Verification items for the finished model (mm, model axes). A direction names the side the tool comes from. Give positions to 0.01 mm unless a question says otherwise; leave off trailing zeros. Loops run counter-clockwise (first coordinate to the right, second up) from the corner with the lowest first, then second, coordinate; pieces in that order, holes last. Notation, with made-up numbers: M -25,-19 L 7,-19 A16 cw 7,7 Z; hole C 53,-38 d9. An arc over 180 degrees is marked long. Put each result on its own line as item: value. Start each with the question number.
from build123d import *

# Parameters (mm, degrees)
SKETCH1_R           = 4.60375
BOSS_EXTRUDE1_DEPTH = 127
SKETCH3_R           = 1.249999967
CUT_EXTRUDE3_DEPTH  = 190.290136172
SKETCH4_R           = 1.1
CUT_EXTRUDE4_DEPTH  = 189.880695817
SKETCH5_W           = 5.08
SKETCH5_H           = 127
BOSS_EXTRUDE2_DEPTH = 50.8
SKETCH6_R           = 0.899999978
CUT_EXTRUDE5_DEPTH  = 5.08
SKETCH7_W           = 6.432611175
SKETCH7_H           = 24.280435839
SKETCH7_W_2         = 25.4
SKETCH7_H_2         = 5.08
SKETCH7_W_3         = 7.534248642
SKETCH7_H_3         = 19.188789511
CUT_EXTRUDE6_DEPTH  = 196.180089282
FILLET1_R           = 5.08
SKETCH8_W           = 43.18
SKETCH8_H           = 7.62
BOSS_EXTRUDE3_DEPTH = 62.23
FILLET2_R           = 5.08


with BuildPart() as part:
    # Sketch1 → Boss-Extrude1 (new body)
    with BuildSketch(Plane.XY):
        with BuildLine():
            Line((-0.467721946, 0.970453027), (-0.467721946, -10.459546973))
            Line((-0.467721946, -10.459546973), (139.232278054, -10.459546973))
            Line((139.232278054, -10.459546973), (139.232278054, 0.970453027))
            ThreePointArc((139.232278054, 0.970453027), (132.882278054, 7.320453027), (126.532278054, 0.970453027))
            Line((126.532278054, 0.970453027), (126.532278054, -5.379546973))
            Line((126.532278054, -5.379546973), (12.232278054, -5.379546973))
            Line((12.232278054, -5.379546973), (12.232278054, 0.970453027))
            ThreePointArc((12.232278054, 0.970453027), (5.882278054, 7.320453027), (-0.467721946, 0.970453027))
        make_face()
        with Locations((5.882278054, 0.970453027)):
            Circle(SKETCH1_R, mode=Mode.SUBTRACT)
        with Locations((132.882278054, 0.970453027)):
            Circle(SKETCH1_R, mode=Mode.SUBTRACT)
    extrude(amount=BOSS_EXTRUDE1_DEPTH)

    # Sketch3 → Cut-Extrude3 (cut, through all)
    with BuildSketch(Plane.XZ.offset(10.459546973)):
        with Locations(Location((101.132278054, 81.883033078, 0), (0, 0, 270))):
            Circle(SKETCH3_R)
        with Locations(Location((43.132278054, 81.883033078, 0), (0, 0, 270))):
            Circle(SKETCH3_R)
        with Locations(Location((43.132278054, 32.883033078, 0), (0, 0, 270))):
            Circle(SKETCH3_R)
        with Locations(Location((101.132278054, 32.883033078, 0), (0, 0, 270))):
            Circle(SKETCH3_R)
    extrude(amount=-CUT_EXTRUDE3_DEPTH, mode=Mode.SUBTRACT)

    # Sketch4 → Cut-Extrude4 (cut, through all)
    with BuildSketch(Plane(origin=(0, -5.379546973, 0), x_dir=(1, 0, 0), z_dir=(0, 1, 0))):
        with Locations(Location((16.877982827, -38.47904026, 0), (0, 0, 270))):
            Circle(SKETCH4_R)
        with Locations(Location((16.877982827, -122.479040154, 0), (0, 0, 270))):
            Circle(SKETCH4_R)
        with Locations(Location((83.377982923, -38.47904026, 0), (0, 0, 270))):
            Circle(SKETCH4_R)
        with Locations(Location((83.377982923, -122.479040154, 0), (0, 0, 270))):
            Circle(SKETCH4_R)
    extrude(amount=-CUT_EXTRUDE4_DEPTH, mode=Mode.SUBTRACT)

    # Sketch5 → Boss-Extrude2 (add)
    with BuildSketch(Plane(origin=(0, -5.379546973, 0), x_dir=(1, 0, 0), z_dir=(0, 1, 0))):
        with Locations((110.022278054, -63.5)):
            Rectangle(SKETCH5_W, SKETCH5_H)
    extrude(amount=BOSS_EXTRUDE2_DEPTH)

    # Sketch6 → Cut-Extrude5 (cut)
    with BuildSketch(Plane.ZY.offset(-107.482278054)):
        with Locations((32.475000074, 6.356452923)):
            Circle(SKETCH6_R)
        with Locations((32.475000074, 41.356453027)):
            Circle(SKETCH6_R)
        with Locations((117.475, 6.356452923)):
            Circle(SKETCH6_R)
        with Locations((117.475, 41.356453027)):
            Circle(SKETCH6_R)
        with Locations((7.475000036, 23.856452975)):
            Circle(SKETCH6_R)
    extrude(amount=-CUT_EXTRUDE5_DEPTH, mode=Mode.SUBTRACT)

    # Sketch7 → Cut-Extrude6 (cut, through all)
    with BuildSketch(Plane(origin=(0, -5.379546973, 0), x_dir=(1, 0, 0), z_dir=(0, 1, 0))):
        with Locations((104.265972467, -17.22021792)):
            Rectangle(SKETCH7_W, SKETCH7_H)
        with Locations((63.863358791, -27.662420978)):
            Rectangle(SKETCH7_W_2, SKETCH7_H_2)
        with Locations((99.048382084, -106.880791012)):
            Rectangle(SKETCH7_W_3, SKETCH7_H_3)
    extrude(amount=-CUT_EXTRUDE6_DEPTH, mode=Mode.SUBTRACT)

    # Fillet1
    fillet1_edges = [part.edges().sort_by_distance(p)[0] for p in [
        (126.532278054, -5.379546973, 63.5),
        (139.232278054, -10.459546973, 63.5),
        (-0.467721946, -10.459546973, 63.5),
        (112.562278054, -5.379546973, 63.5),
    ]]
    fillet(fillet1_edges, radius=FILLET1_R)

    # Sketch8 → Boss-Extrude3 (add)
    with BuildSketch(Plane(origin=(0, -5.379546973, 0), x_dir=(1, 0, 0), z_dir=(0, 1, 0))):
        with Locations((54.059666879, -3.81)):
            Rectangle(SKETCH8_W, SKETCH8_H)
    extrude(amount=BOSS_EXTRUDE3_DEPTH)

    # Fillet2
    fillet2_edges = [part.edges().sort_by_distance(p)[0] for p in [
        (32.469666879, -5.379546973, 3.81),
        (75.649666879, -5.379546973, 3.81),
    ]]
    fillet(fillet2_edges, radius=FILLET2_R)


solid = part.part
Q1. Cross-section at C-C, the plane x = 68. Record the boundary of the cut face in (y, z), then the cut area to 3 significant figures.
Q2. Set-up check for faces 4 (the face through (137.273, 2.353, 62.611)), 5 (the face through (101.05, -8, 17)), 6 (the face through (54, 25, 7.62)), 7 (the face through (125.084, -3.852, 64.389)): record each of +Z, -Z, +X, -X, +Y, -Y from which the full face is reachable in a straight line by a thin tool's end or side.
Q3. Go/stop test with flat-tipped pins: pin 1 (4 mm diameter, centred on x = 65, y = -9, fed in from -Z); pin 2 (2.5 mm diameter, centred on y = 15.5, z = 2.5, fed in from +X); pin 3 (1.5 mm diameter, centred on x = 101.13, z = 81.88, fed in from -Y); pin 4 (5.5 mm diameter, centred on y = -9, z = 28.5, fed in from -X). Record where each tip stops, or that it passes through.
Q4. Cross-section at A-A, the plane z = 101.5. Record the boundary of the cut face in (x, y).
Q5. Scan lines: L1, parallel to X at y = -1, z = 15; L2, parallel to Y at x = 74.5, z = 74; L3, parallel to X at y = 44.5, z = 57. Record each from-to range of solid material in increasing order.
Q6. Release check for a two-part mould opening along X. For faces 1 (the face through (77.177, -3.931, 3.757)), 2 (the face through (68, -10.46, 63)), 3 (the face through (137.705, -9.011, 64.389)) record: pulls with the +X half, pulls with the -X half, needs draft (parallel to the pull), parting line crosses it, or undercut.
Q7. Cross-section at D-D, the plane z = 53. Record the boundary of the cut face in (x, y), then the cut area to 3 significant figures.
Q8. Cross-section at B-B, the plane y = 33. Record the boundary of the cut face in (x, z).
Ans:
1. outline: M -10.46,0 L 56.85,0 L 56.85,7.62 L -5.38,7.62 L -5.38,25.12 L -10.46,25.12 Z; M -10.46,30.2 L -5.38,30.2 L -5.38,127 L -10.46,127 Z
1. area: 1,090 mm^2
2. face 4: +Z, -Z
2. face 5: +Y, -Y
2. face 6: +Z, +Y
2. face 7: +Z, -Z, +Y
3. pin 1: stops at z = 0
3. pin 2: stops at x = 112.56
3. pin 3: passes through
3. pin 4: stops at x = -0.39
4. outline: M -0.47,-5.38 A5.08 ccw 4.61,-10.46 L 95.28,-10.46 L 95.28,-5.38 L 12.23,-5.38 L 12.23,0.97 A6.35 ccw -0.47,0.97 Z; M 102.82,-10.46 L 134.15,-10.46 A5.08 ccw 139.23,-5.38 L 139.23,0.97 A6.35 ccw 126.53,0.97 L 126.53,-0.3 A5.08 cw 121.45,-5.38 L 117.64,-5.38 A5.08 cw 112.56,-0.3 L 112.56,45.42 L 107.48,45.42 L 107.48,-5.38 L 102.82,-5.38 Z; hole C 5.88,0.97 d9.21; hole C 132.88,0.97 d9.21
5. L1: x = -0.47 to 1.72, 10.04 to 12.23, 107.48 to 112.61, 126.48 to 128.72, 137.04 to 139.23
5. L2: y = -10.46 to -5.38
5. L3: x = 107.48 to 112.56
6. face 1: undercut
6. face 2: needs draft
6. face 3: pulls with the +X half
7. outline: M -0.47,-5.38 A5.08 ccw 4.61,-10.46 L 134.15,-10.46 A5.08 ccw 139.23,-5.38 L 139.23,0.97 A6.35 ccw 126.53,0.97 L 126.53,-0.3 A5.08 cw 121.45,-5.38 L 117.64,-5.38 A5.08 cw 112.56,-0.3 L 112.56,45.42 L 107.48,45.42 L 107.48,-5.38 L 12.23,-5.38 L 12.23,0.97 A6.35 ccw -0.47,0.97 Z; hole C 5.88,0.97 d9.21; hole C 132.88,0.97 d9.21
7. area: 1,120 mm^2
8. outline: M 32.47,0 L 75.65,0 L 75.65,7.62 L 32.47,7.62 Z; M 107.48,0 L 112.56,0 L 112.56,127 L 107.48,127 Z
